```python
from build123d import *

# Parameters (mm, degrees)
SKETCH2_R           = 6.1
BOSS_EXTRUDE1_DEPTH = 6.5
SKETCH3_R           = 0.325
BOSS_EXTRUDE2_DEPTH = 15
FILLET1_R           = 1


with BuildPart() as part:
    # Sketch2 → Boss-Extrude1 (new body)
    with BuildSketch(Plane(origin=(0, 0, 0), x_dir=(1, 0, 0), z_dir=(0, 1, 0))):
        with Locations(Location((0, 0, 0), (0, 0, 90))):
            Circle(SKETCH2_R)
    extrude(amount=BOSS_EXTRUDE1_DEPTH)

    # Sketch3 → Boss-Extrude2 (add)
    with BuildSketch(Plane.XZ):
        with Locations(Location((-2.5, 0, 0), (0, 0, 90))):
            Circle(SKETCH3_R)
        with Locations(Location((2.5, 0, 0), (0, 0, 90))):
            Circle(SKETCH3_R)
    extrude(amount=BOSS_EXTRUDE2_DEPTH)

    # Fillet1
    fillet1_edges = [part.edges().sort_by_distance(p)[0] for p in [
        (0, 6.5, 6.1),
    ]]
    fillet(fillet1_edges, radius=FILLET1_R)


solid = part.part
```
Could you check a few things on this model? Use its own coordinates, in mm. Coordinates: 2 decimals unless noted, no trailing zeros. Write each loop counter-clockwise with the first axis right and the second up, starting at its lowest first coordinate (ties: lowest second). Pieces come first, ordered by that corner, then holes. Notation, with made-up numbers: (56, -7.5) -> (106, -7.5) arc R25 ccw to (106, 14.5) -> close; hole circle Ø6 at (57, -30). An arc over 180 degrees is marked (long way). Write item = value, one per line. Start each with the question number.
(1) I want a section at D-D (y = 2.5). Please give me the cut outline in (x, z).
(2) I need wall thicknesses on line 1 (Y direction, x = 2, z = 3); line 2 (X direction, y = 3.5, z = -3.25); line 3 (Z direction, x = -3.5, y = 1.75). Which ranges of each line are inside material? Lowest first, please. Write a range as [from, to].
(3) Will these pins go through, and if not, where does the flat tip stop? pin 1 (3 mm diameter, centred on y = -8, z = 2.5, fed in from +X); pin 2 (4 mm diameter, centred on y = -10.5, z = 1, fed in from +X) (3 decimals); pin 3 (2 mm diameter, centred on x = -2.5, y = -11, fed in from +Z) (3 decimals).
(4) I want a section at A-A (y = -11.5). Please give me the cut outline in (x, z) (3 decimals), plus the area to 3 significant figures.
(5) I want a section at C-C (x = 0). Please give me the cut outline in (y, z), plus the area to 3 significant figures.
(6) I want a section at B-B (z = 0). Please give me the cut outline in (x, y) (3 decimals).
Result set:
q1.outline = circle Ø12.2 at (0, 0)
q2.line_1 = [0, 6.5]
q2.line_2 = [-5.16, 5.16]
q2.line_3 = [-5, 5]
q3.pin_1 = through
q3.pin_2 = 2.825
q3.pin_3 = 0.325
q4.outline = circle Ø0.65 at (-2.5, 0); circle Ø0.65 at (2.5, 0)
q4.area = 0.664 mm2
q5.outline = (0, -6.1) -> (5.5, -6.1) arc R1 ccw to (6.5, -5.1) -> (6.5, 5.1) arc R1 ccw to (5.5, 6.1) -> (0, 6.1) -> close
q5.area = 78.9 mm2
q6.outline = (-6.1, 0) -> (-2.825, 0) -> (-2.825, -15) -> (-2.175, -15) -> (-2.175, 0) -> (2.175, 0) -> (2.175, -15) -> (2.825, -15) -> (2.825, 0) -> (6.1, 0) -> (6.1, 5.5) arc R1 ccw to (5.1, 6.5) -> (-5.1, 6.5) arc R1 ccw to (-6.1, 5.5) -> close
